Could you check a few things on this model? Use its own coordinates, in mm. Face numbers are marked on the shaded views. A direction names the side the tool comes from. Give positions to 0.01 mm unless a question says otherwise; leave off trailing zeros. Loops run counter-clockwise (first coordinate to the right, second up) from the corner with the lowest first, then second, coordinate; pieces in that order, holes last. Notation, with made-up numbers: (52.5, 79.25) - (96.5, 79.25) arc R19 cw to (96.5, 101.25) - close; hole circle Ø4 at (17.25, 44.5). An arc over 180 degrees is marked (long way). Answer in a Markdown table with one row per item. Add a question column.
```python
from build123d import *

# Parameters (mm, degrees)
SKETCH_1_R          = 15
EXTRUDE_1_DEPTH     = 4
SKETCH_3_R          = 14
CUT_EXTRUDE_2_DEPTH = 2
SKETCH_5_R          = 3
CUT_EXTRUDE_3_DEPTH = 3
CHAMFER_1_SIZE      = 0.5
CHAMFER_3_SIZE      = 0.5


with BuildPart() as part:
    # Эскиз1 → Вытянуть1 (new body)
    with BuildSketch(Plane.XY):
        Circle(SKETCH_1_R)
    extrude(amount=EXTRUDE_1_DEPTH)

    # Эскиз3 → Вытянуть2 (cut)
    with BuildSketch(Plane(origin=(0, 0, 0), x_dir=(-1, 0, 0), z_dir=(0, 0, -1))):
        Circle(SKETCH_3_R)
    extrude(amount=-CUT_EXTRUDE_2_DEPTH, mode=Mode.SUBTRACT)

    # Эскиз5 → Вытянуть3 (cut, through all)
    with BuildSketch(Plane(origin=(0, 0, 2), x_dir=(-1, 0, 0), z_dir=(0, 0, -1))):
        with Locations((9.998142701, 0.192724)):
            Circle(SKETCH_5_R)
        with Locations((-0.192724, -9.998142701)):
            Circle(SKETCH_5_R)
        with Locations((0.1908667, 10)):
            Circle(SKETCH_5_R)
        with Locations((-10, -0.1908667)):
            Circle(SKETCH_5_R)
    extrude(amount=-CUT_EXTRUDE_3_DEPTH, mode=Mode.SUBTRACT)

    # Фаска1
    chamfer_1_edges = [part.edges().sort_by_distance(p)[0] for p in [
        (-15, 0, 4),
    ]]
    chamfer(chamfer_1_edges, length=CHAMFER_1_SIZE)

    # Фаска3
    chamfer_3_edges = [part.edges().sort_by_distance(p)[0] for p in [
        (-15, 0, 0),
    ]]
    chamfer(chamfer_3_edges, length=CHAMFER_3_SIZE)


solid = part.part
```
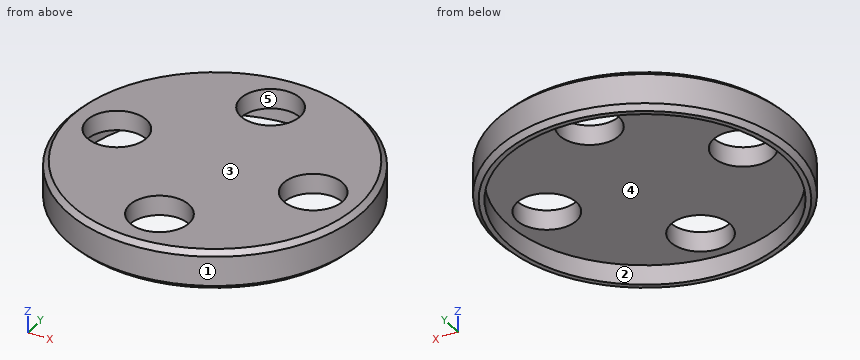
(1) I want a section at A-A on x = 0. Please give me the cut outline in (y, z).
(2) On a 3-axis mill with a long thin cutter (end or side, diameter ignored), from which of +Z, -Z, +X, -X, +Y, -Y can I reach the whole of each face in a straight line? I mean the marked faces 4 and 5. Say none if no direction works.
(3) For pin 1 Ø8 at (x, y) = (-3, -3) entering from -Z; pin 2 Ø1 at (x, z) = (8, 2.5) entering from -Y; pin 3 Ø1 at (x, z) = (-10.5, 1) entering from +Y, each with a flat end and sliding along its axis, tell me the tip position at first contact or that it passes through.
(4) Please list where these lines run through material, in increasing order: line 1 (Y direction, x = 0, z = 0.5); line 2 (X direction, y = -2.5, z = 2.65); line 3 (Y direction, x = -1.5, z = 2.3).
(5) I want a section at C-C on y = -0.75. State how many separate pieces and enclosed holes the cut face has, then the cut area to 3 significant figures.
(6) We'd pull the mould along Y, two halves only. Please class the marked faces 1, 2 and 3: pulls with the +Y half, pulls with the -Y half, needs draft (parallel to the pull), parting line crosses it, or undercut.
(7) I want a section at B-B on z = 1. Please give me the cut outline in (x, y), then the cut area to 3 significant figures.
Reported:
| question | item | result |
|---|---|---|
| 1 | outline | (-15, 0.5) - (-14.5, 0) - (-14, 0) - (-14, 2) - (-12.99, 2) - (-12.99, 4) - (-14.5, 4) - (-15, 3.5) - close; (-7, 2) - (7.01, 2) - (7.01, 4) - (-7, 4) - close; (12.99, 2) - (14, 2) - (14, 0) - (14.5, 0) - (15, 0.5) - (15, 3.5) - (14.5, 4) - (12.99, 4) - close |
| 2 | face 4 | -Z |
| 2 | face 5 | +Z, -Z |
| 3 | pin 1 | z = 2 |
| 3 | pin 2 | y = -12.99 |
| 3 | pin 3 | y = 11.18 |
| 4 | line 1 | -15 to -14, 14 to 15 |
| 4 | line 2 | -14.79 to -11.32, -8.68 to 8.08, 11.92 to 14.79 |
| 4 | line 3 | -14.92 to -12.47, -7.52 to 7.3, 12.7 to 14.92 |
| 5 | separate pieces | 3 |
| 5 | enclosed holes | 0 |
| 5 | area | 40.2 mm² |
| 6 | face 1 | parting line crosses it |
| 6 | face 2 | undercut |
| 6 | face 3 | needs draft |
| 7 | outline | circle Ø30 at (0, 0); hole circle Ø28 at (0, 0) |
| 7 | area | 91.1 mm² |
